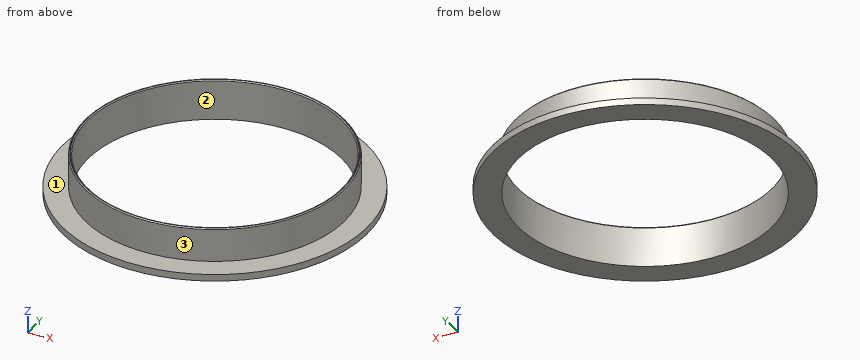
```python
from build123d import *

# Parameters (mm, degrees)
SKETCH_R        = 45
SKETCH_R_2      = 37.5
PAD_DEPTH       = 2
SKETCH001_R     = 38.3
SKETCH001_R_2   = 37.5
PAD001_DEPTH    = 10
CHAMFER_SIZE    = 0.3
CHAMFER001_SIZE = 0.3


with BuildPart() as part:
    # Sketch → Pad (new body)
    with BuildSketch(Plane.XY):
        Circle(SKETCH_R)
        Circle(SKETCH_R_2, mode=Mode.SUBTRACT)
    extrude(amount=PAD_DEPTH)

    # Sketch001 (on Face4 of Pad) → Pad001 (join)
    with BuildSketch(Plane.XY.offset(2)):
        Circle(SKETCH001_R)
        Circle(SKETCH001_R_2, mode=Mode.SUBTRACT)
    extrude(amount=PAD001_DEPTH)

    # Chamfer
    chamfer_edges = [part.edges().sort_by_distance(p)[0] for p in [
        (-37.5, 0, 12),
    ]]
    chamfer(chamfer_edges, length=CHAMFER_SIZE)

    # Chamfer001
    chamfer001_edges = [part.edges().sort_by_distance(p)[0] for p in [
        (-38.3, 0, 12),
    ]]
    chamfer(chamfer001_edges, length=CHAMFER001_SIZE)


solid = part.part
```
For this review, take the finished solid that the model builds, in its own axes (mm). Face numbers are marked on the shaded views. Round coordinates to 2 decimals unless told otherwise and drop trailing zeros. Order: outer loops, then holes, each group sorted by start corner. A loop starts at its lowest first (then second) coordinate and runs counter-clockwise, first axis right, second up. Notation, with made-up numbers: (12.25, -19) -> (63.25, -19) arc R22 cw to (63.25, -1) -> close; hole circle Ø11 at (-28, 44.25). An arc over 180 degrees is marked (long way). Use a Markdown table: item, result.
Item 1: For pin 1 (4 mm diameter, centred on x = 14.5, z = 1.5, fed in from -Y); pin 2 (1.5 mm diameter, centred on x = 4.5, z = 4.5, fed in from +Y); pin 3 (1.5 mm diameter, centred on y = -13.5, z = 4, fed in from +X), all flat-tipped, find the tip position at first contact; note any pin that passes through.
Resolved:
| item | result |
|---|---|
| pin 1 | stops at y = -43.23 |
| pin 2 | stops at y = 38.12 |
| pin 3 | stops at x = 36.12 |
Item 2: For line 1 along Y through (x, z) = (0, 9); line 2 along Y through (x, z) = (30, 8.5); line 3 along X through (y, z) = (3, 0.5), list the stretches that pass through material, from the lowest coordinate up. Write a range as [from, to].
Resolved:
| item | result |
|---|---|
| line 1 | y = [-38.3, -37.5], [37.5, 38.3] |
| line 2 | y = [-23.81, -22.5], [22.5, 23.81] |
| line 3 | x = [-44.9, -37.38], [37.38, 44.9] |
Item 3: Draft analysis for pull direction Y (two halves, no side actions). For the marked faces 1, 2 and 3, state which applies: +Y half, -Y half, draft (parallel to the pull), parting line (faces both ways), or undercut.
Resolved:
| item | result |
|---|---|
| face 1 | draft |
| face 2 | undercut |
| face 3 | parting line |
Item 4: Take a section at A-A (y = 0). State the section outline as (x, z) points.
Resolved:
| item | result |
|---|---|
| outline | (-45, 0) -> (-37.5, 0) -> (-37.5, 11.7) -> (-37.8, 12) -> (-38, 12) -> (-38.3, 11.7) -> (-38.3, 2) -> (-45, 2) -> close; (37.5, 0) -> (45, 0) -> (45, 2) -> (38.3, 2) -> (38.3, 11.7) -> (38, 12) -> (37.8, 12) -> (37.5, 11.7) -> close |
Item 5: Take a section at C-C (z = 9). State the section outline as (x, y) points, plus the area to 3 significant figures.
Resolved:
| item | result |
|---|---|
| outline | circle Ø76.6 at (0, 0); hole circle Ø75 at (0, 0) |
| area | 191 mm² |
